The model under review builds one solid part; all positions refer to its coordinate system, in mm. Coordinates: 2 decimals unless noted, no trailing zeros. Write each loop counter-clockwise with the first axis right and the second up, starting at its lowest first coordinate (ties: lowest second). Pieces come first, ordered by that corner, then holes.
Autodesk Fusion 360 part; units mm, degrees
sketch "Sketch1" plane through (0, 0, 0) normal (0, 0, 1) x (1, 0, 0)
  line L0 (0, 0) -> (40, 0)
  line L1 (40, 0) -> (40, -20)
  line L2 (40, -20) -> (0, -20)
  line L3 (0, -20) -> (0, 0)
sketch "Sketch2" plane through (0, 0, 0) normal (0, 1, 0) x (1, 0, 0)
  line L0 (0, 0) -> (20, 0)
  line L1 (20, 0) -> (20, 40)
  line L2 (20, 40) -> (0, 40)
  line L3 (0, 40) -> (0, 0)
extrude "Extrude2" add sketch "Sketch2" along normal blind 10
hole "Hole1" at (10, 10, -20) direction (0, -1, 0) diameter 5 depth 10 tip angle 118
fillet "Fillet1" radius 2 1 edges at (20, 5, 0)
fillet "Fillet2" radius 2 1 edges at (0, 5, 0)
fillet "Fillet3" radius 2 1 edges at (0, 5, -40)
fillet "Fillet4" radius 2 1 edges at (20, 5, -40)
Item 1: Mouldability with a two-part tool opening along Z and no side actions: class faces 1 (the face through (19.43, 5.07, -39.4)), 2 (the face through (0, 5, -20)), 3 (the face through (10, 5, 0)), 4 (the face through (11.5, 4.9, -22)) as pulls with the +Z half, pulls with the -Z half, needs draft (parallel to the pull), parting line crosses it, or undercut.
Solved:
face 1: pulls with the -Z half
face 2: needs draft
face 3: pulls with the +Z half
face 4: undercut
Item 2: Take a section at B-B, the plane z = -20. Write out the cut boundary in (x, y).
Solved:
outline: (0, 0) - (7.5, 0) - (7.5, 10) - (0, 10) - close; (12.5, 0) - (20, 0) - (20, 10) - (12.5, 10) - close
Item 3: For pin 1 (1.5 mm diameter, centred on y = 8.5, z = -22, fed in from -X), flat-tipped, find the tip position at first contact; note if it passes through.
Solved:
pin 1: stops at x = 0
Item 4: To check wall thickness, follow line 1 along Z through (x, y) = (10, 6.5); line 2 along X through (y, z) = (2, -20); line 3 along Z through (x, y) = (9.25, 7.75). State the ranges of each line that lie inside material, in increasing order.
Solved:
line 1: z = -40 to -22.5, -17.5 to 0
line 2: x = 0 to 7.5, 12.5 to 20
line 3: z = -40 to -22.38, -17.62 to 0
Item 5: Take a section at C-C, the plane y = 6. Write out the cut boundary in (x, z).
Solved:
outline: (0, -38) arc R2 ccw to (2, -40) - (18, -40) arc R2 ccw to (20, -38) - (20, -2) arc R2 ccw to (18, 0) - (2, 0) arc R2 ccw to (0, -2) - close; hole circle Ø5 at (10, -20)
Item 6: Take a section at A-A, the plane x = 12. Write out the cut boundary in (y, z).
Solved:
outline: (0, -40) - (10, -40) - (10, -21.5) - (0, -21.5) - close; (0, -18.5) - (10, -18.5) - (10, 0) - (0, 0) - close
